Verification items for this drawing (mm, ordinates from the low corner). A direction names the side the tool comes from. Give positions to 0.01 mm unless a question says otherwise; leave off trailing zeros. Loops run counter-clockwise (first coordinate to the right, second up) from the corner with the lowest first, then second, coordinate; pieces in that order, holes last. Notation, with made-up numbers: (-1, 46.5) -> (38, 46.5) arc R16 ccw to (38, 54.5) -> close; hole circle Ø10 at (-29.5, 79.25). An arc over 180 degrees is marked (long way). Answer as CSV lines item,"result". Start each with the question number.
(1) Access from +Z, -Z, +X, -X, +Y, -Y to the whole of each face (thin tool, end or side, straight path). Record for the marked faces 1 and 2.
(2) Section check B-B on z = 11. Enter the section's corners in (x, y), plus the area to 3 significant figures.
(3) Gauge pin test, flat ends, axial feed: pin 1 Ø8 at (y, z) = (11.5, 30) entering from +X; pin 2 Ø5 at (x, y) = (30.5, 14.5) entering from -Z; pin 3 Ø4 at (x, y) = (3.5, 3) entering from -Z. Record the tip position at first contact, or that the pin passes through.
(4) Section check D-D on x = 24. Enter the section's corners in (y, z), plus the area to 3 significant figures.
(5) Section check C-C on y = 7. Enter the section's corners in (x, z) (3 decimals).
(6) Section check A-A on x = 18. Enter the section's corners in (y, z) (1 decimal).
(7) Material ranges on line 1 (X direction, y = 5, z = 17.5); line 2 (Z direction, x = 16.5, y = 7); line 3 (Y direction, x = 7, z = 13), recorded low to high. Write a range as from..to.
(8) Release check for a two-part mould opening along X. For the marked faces 3, 4 and 5 record: pulls with the +X half, pulls with the -X half, needs draft (parallel to the pull), parting line crosses it, or undercut.
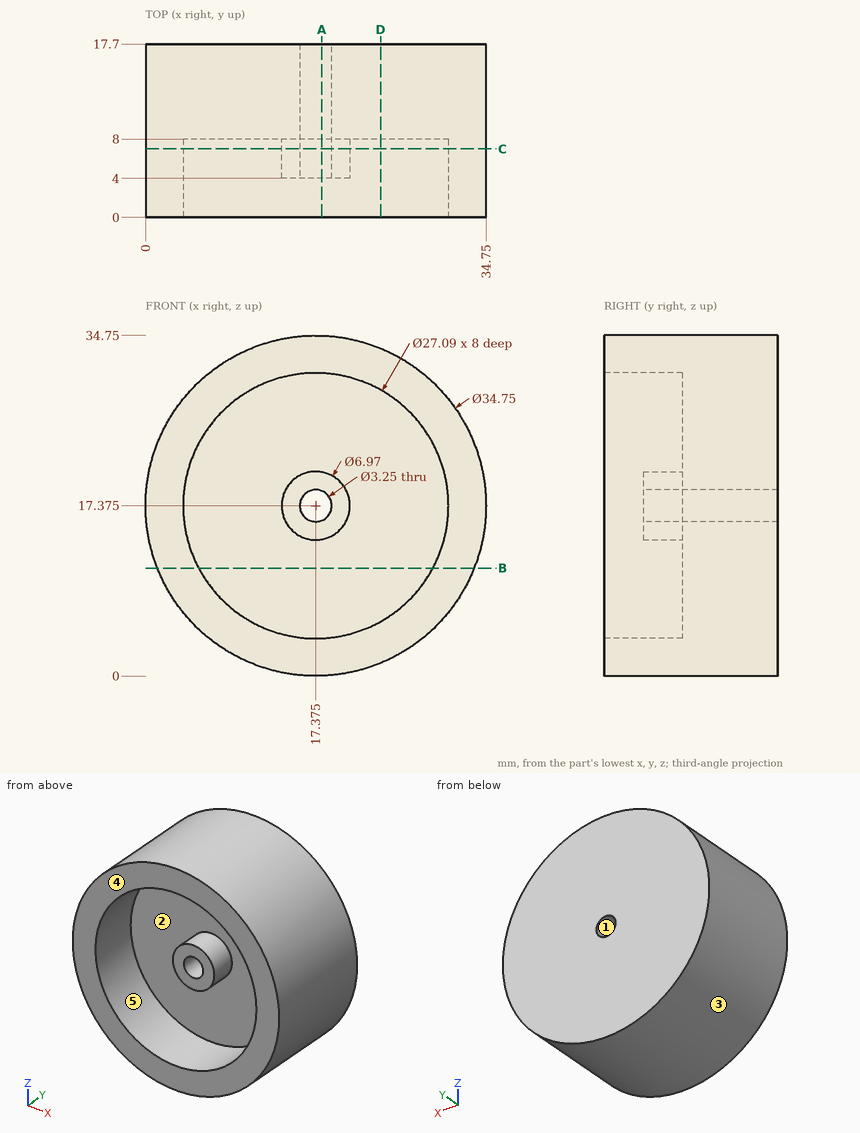
Working result:
1,face 1,"+Y, -Y"
1,face 2,"-Y"
2,outline,"(1.21, 0) -> (5.42, 0) -> (5.42, 8) -> (29.33, 8) -> (29.33, 0) -> (33.54, 0) -> (33.54, 17.7) -> (1.21, 17.7) -> close"
2,area,"381 mm^2"
3,pin 1,"stops at x = 32.46"
3,pin 2,"stops at z = 3.63"
3,pin 3,"stops at z = 4.69"
4,outline,"(0, 1.31) -> (17.7, 1.31) -> (17.7, 33.44) -> (0, 33.44) -> (0, 29.19) -> (8, 29.19) -> (8, 5.56) -> (0, 5.56) -> close"
4,area,"380 mm^2"
5,outline,"circle Ø34.75 at (17.375, 17.375); circle Ø6.97 at (17.375, 17.375); hole circle Ø27.09 at (17.375, 17.375); hole circle Ø3.25 at (17.375, 17.375)"
6,outline,"(0, 0) -> (17.7, 0) -> (17.7, 15.9) -> (4, 15.9) -> (4, 13.9) -> (8, 13.9) -> (8, 3.8) -> (0, 3.8) -> close; (0, 30.9) -> (8, 30.9) -> (8, 20.8) -> (4, 20.8) -> (4, 18.9) -> (17.7, 18.9) -> (17.7, 34.7) -> (0, 34.7) -> close"
7,line 1,"x = 0..3.83, 13.89..15.75, 19..20.86, 30.92..34.75"
7,line 2,"z = 0.02..3.86, 14..16.01, 18.74..20.75, 30.89..34.73"
7,line 3,"y = 8..17.7"
8,face 3,"parting line crosses it"
8,face 4,"needs draft"
8,face 5,"undercut"
